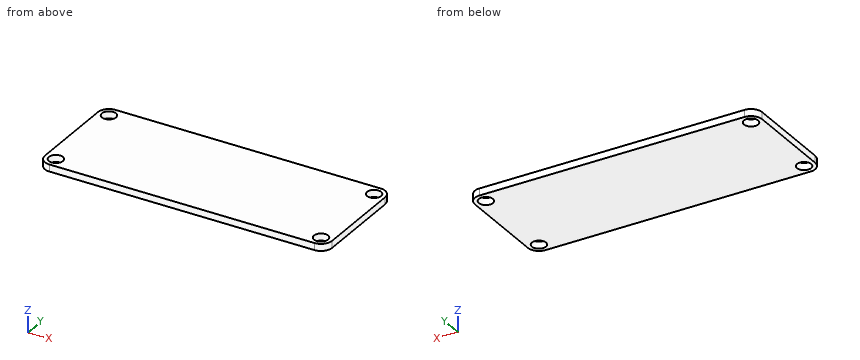
Autodesk Inventor part; units mm, degrees
ref_plane "YZ Plane" through (0, 0, 0) normal (1, 0, 0) x (0, 1, 0)
ref_plane "XZ Plane" through (0, 0, 0) normal (0, 1, 0) x (-1, 0, 0)
ref_plane "XY Plane" through (0, 0, 0) normal (0, 0, 1) x (1, 0, 0)
sketch "Sketch1" plane through (0, 0, 0) normal (0, 0, 1) x (1, 0, 0)
  line L0 (0, 0) -> (82.55, 0)
  line L1 (82.55, 0) -> (82.55, 31.75)
  line L2 (82.55, 31.75) -> (0, 31.75)
  line L3 (0, 31.75) -> (0, 0)
  dimension "d0" = 82.55
  dimension "d1" = 31.75
extrude "Extrusion1" add sketch "Sketch1" along normal blind 2
fillet "Fillet1" radius 3.175 1 edges at (0, 31.75, 1)
fillet "Fillet2" radius 3.175 1 edges at (82.55, 31.75, 1)
fillet "Fillet3" radius 3.175 1 edges at (82.55, 0, 1)
fillet "Fillet4" radius 3.175 1 edges at (0, 0, 1)
sketch "Sketch2" plane through (0, 0, 2) normal (0, 0, 1) x (1, 0, 0)
  circle A0 centre (3.175, 3.175) radius 2.032
  arc A1 (0, 3.175) -> (3.175, 0) centre (3.175, 3.175) ccw
  line L0 (3.175, 0) -> (79.375, 0)
  arc A2 (79.375, 0) -> (82.55, 3.175) centre (79.375, 3.175) ccw
  line L1 (82.55, 3.175) -> (82.55, 28.575)
  arc A3 (82.55, 28.575) -> (79.375, 31.75) centre (79.375, 28.575) ccw
  line L2 (79.375, 31.75) -> (3.175, 31.75)
  arc A4 (3.175, 31.75) -> (0, 28.575) centre (3.175, 28.575) ccw
  line L3 (0, 28.575) -> (0, 3.175)
  point P0 (0, 0)
  dimension "d8" = 4.064
  dimension "d23" = 25.4
  dimension "d25" = 76.2
hole "Hole1" at (3.175, 3.175, 2) direction (0, 0, -1) diameter 4.064 end through all
sketch "Sketch7" plane through (0, 0, 2) normal (0, 0, 1) x (1, 0, 0)
  circle A0 centre (3.175, 3.175) radius 2.032
  circle A1 centre (3.175, 3.175) radius 2.032
  arc A2 (0, 3.175) -> (3.175, 0) centre (3.175, 3.175) ccw
  line L0 (3.175, 0) -> (79.375, 0)
  arc A3 (79.375, 0) -> (82.55, 3.175) centre (79.375, 3.175) ccw
  line L1 (82.55, 3.175) -> (82.55, 28.575)
  arc A4 (82.55, 28.575) -> (79.375, 31.75) centre (79.375, 28.575) ccw
  line L2 (79.375, 31.75) -> (3.175, 31.75)
  arc A5 (3.175, 31.75) -> (0, 28.575) centre (3.175, 28.575) ccw
  line L3 (0, 28.575) -> (0, 3.175)
  circle A6 centre (3.175, 28.575) radius 2.032
  point P0 (0, 0)
  dimension "d28" = 4.064
hole "Hole2" at (3.175, 28.575, 2) direction (0, 0, -1) diameter 4.064 end through all
sketch "Sketch8" plane through (0, 0, 2) normal (0, 0, 1) x (1, 0, 0)
  circle A0 centre (3.175, 3.175) radius 2.032
  circle A1 centre (3.175, 28.575) radius 2.032
  circle A2 centre (3.175, 3.175) radius 2.032
  arc A3 (0, 3.175) -> (3.175, 0) centre (3.175, 3.175) ccw
  line L0 (3.175, 0) -> (79.375, 0)
  arc A4 (79.375, 0) -> (82.55, 3.175) centre (79.375, 3.175) ccw
  line L1 (82.55, 3.175) -> (82.55, 28.575)
  arc A5 (82.55, 28.575) -> (79.375, 31.75) centre (79.375, 28.575) ccw
  line L2 (79.375, 31.75) -> (3.175, 31.75)
  arc A6 (3.175, 31.75) -> (0, 28.575) centre (3.175, 28.575) ccw
  line L3 (0, 28.575) -> (0, 3.175)
  circle A7 centre (79.375, 28.575) radius 2.032
  point P0 (0, 0)
  dimension "d36" = 4.064
hole "Hole3" at (79.375, 28.575, 2) direction (0, 0, -1) diameter 4.064 end through all
sketch "Sketch9" plane through (0, 0, 2) normal (0, 0, 1) x (1, 0, 0)
  circle A0 centre (3.175, 3.175) radius 2.032
  circle A1 centre (79.375, 28.575) radius 2.032
  circle A2 centre (3.175, 28.575) radius 2.032
  circle A3 centre (3.175, 3.175) radius 2.032
  arc A4 (0, 3.175) -> (3.175, 0) centre (3.175, 3.175) ccw
  line L0 (3.175, 0) -> (79.375, 0)
  arc A5 (79.375, 0) -> (82.55, 3.175) centre (79.375, 3.175) ccw
  line L1 (82.55, 3.175) -> (82.55, 28.575)
  arc A6 (82.55, 28.575) -> (79.375, 31.75) centre (79.375, 28.575) ccw
  line L2 (79.375, 31.75) -> (3.175, 31.75)
  arc A7 (3.175, 31.75) -> (0, 28.575) centre (3.175, 28.575) ccw
  line L3 (0, 28.575) -> (0, 3.175)
  circle A8 centre (79.375, 3.175) radius 2.032
  point P0 (0, 0)
  dimension "d44" = 4.064
hole "Hole4" at (79.375, 3.175, 2) direction (0, 0, -1) diameter 4.064 end through all
properties part number "I6ABreakout"
Input: part model. Units: mm. Frame: model coordinates. Round coordinates to 2 decimals unless told otherwise and drop trailing zeros. Write each loop counter-clockwise with the first axis right and the second up, starting at its lowest first coordinate (ties: lowest second). Pieces come first, ordered by that corner, then holes. Notation, with made-up numbers: (15.25, -7) -> (21.25, -7) arc R9 cw to (21.25, -1) -> close; hole circle Ø1 at (34.5, 54). An arc over 180 degrees is marked (long way). Answer as CSV lines item,"result".
1. Contact query for a flat-ended pin moving along its axis: P1, Ø3.5, axis at x = 79.375, y = 28.575, coming from the -Z side. Output: stop coordinate, or through.
Geometry says:
P1,"passes through"
2. Section A-A (z = 0.65). Return the cut outline in (x, y) (3 decimals), plus the area to 3 significant figures.
Geometry says:
outline,"(0, 3.175) arc R3.175 ccw to (3.175, 0) -> (79.375, 0) arc R3.175 ccw to (82.55, 3.175) -> (82.55, 28.575) arc R3.175 ccw to (79.375, 31.75) -> (3.175, 31.75) arc R3.175 ccw to (0, 28.575) -> close; hole circle Ø4.064 at (3.175, 3.175); hole circle Ø4.064 at (3.175, 28.575); hole circle Ø4.064 at (79.375, 3.175); hole circle Ø4.064 at (79.375, 28.575)"
area,"2,560 mm^2"
3. Ray query, L1, parallel to X at y = 28.5, z = 0.8; L2, parallel to X at y = 27, z = 0.9. Return the intervals inside material, ascending. Write a range as [from, to].
Geometry says:
L1,"x = [0, 1.14], [5.21, 77.34], [81.41, 82.55]"
L2,"x = [0, 1.89], [4.46, 78.09], [80.66, 82.55]"
